Autodesk Inventor part; units mm, degrees
ref_plane "YZ Plane" through (0, 0, 0) normal (1, 0, 0) x (0, 1, 0)
ref_plane "XZ Plane" through (0, 0, 0) normal (0, 1, 0) x (-1, 0, 0)
ref_plane "XY Plane" through (0, 0, 0) normal (0, 0, 1) x (1, 0, 0)
sketch "Sketch1" plane through (0, 0, 0) normal (0, 1, 0) x (-1, 0, 0)
  line L0 (10, -18.5) -> (-10, -18.5)
  line L1 (-10, -18.5) -> (-10, 18.5)
  line L2 (-10, 18.5) -> (10, 18.5)
  line L3 (10, 18.5) -> (10, -18.5)
  point P0 (0, 0)
  dimension "d0" = 20
  dimension "d1" = 37
  dimension "d2" = 18.5
  dimension "d3" = 10
extrude "Plate1" add sketch "Sketch1" along normal blind 1.5
sketch "Sketch2" plane through (-10, 0, -20) normal (0, 0, 1) x (1, 0, 0)
  line L0 (20, 0) -> (0, 0)
  line L1 (0, 0) -> (0, 31.5)
  line L2 (0, 31.5) -> (20, 31.5)
  line L3 (20, 31.5) -> (20, 0)
edge flange "Flange1" height 31.5 angle 90 thickness 1.5 bend radius 0.31 thickness toward (0, 0, 1) relief tear relief width 1.5 relief depth 0.75 edges at (0, 1.5, -18.5) wall of the first edge with corners at (10, 0, -20) (-10, 0, -20) (-10, 31.5, -20) (10, 31.5, -20)
bend "Bend1"
corner "Corner1"
sketch "Sketch3" plane through (10, 0, 20) normal (0, 0, -1) x (-1, 0, 0)
  line L0 (20, 0) -> (0, 0)
  line L1 (0, 0) -> (0, 51.5)
  line L2 (0, 51.5) -> (20, 51.5)
  line L3 (20, 51.5) -> (20, 0)
edge flange "Flange2" height 51.5 angle 90 thickness 1.5 bend radius 0.31 thickness toward (0, 0, -1) relief tear relief width 1.5 relief depth 0.75 edges at (0, 1.5, 18.5) wall of the first edge with corners at (-10, 0, 20) (10, 0, 20) (10, 51.5, 20) (-10, 51.5, 20)
bend "Bend2"
corner "Corner2"
sketch "Sketch4" plane through (-10, 51.5, 20) normal (0, 0, 1) x (1, 0, 0)
  circle A0 centre (10, -10) radius 10
  line L0 (0, 0) -> (20, 0)
  line L1 (0, 0) -> (20, 0)
  line L2 (20, 0) -> (20, -10)
  line L3 (20, -10) -> (0, -10)
  line L4 (0, -10) -> (0, 0)
  line L5 (0, -49.69) -> (0, 0)
  point P0 (10, -51.5)
  point P1 (10, 0)
  dimension "d26" = 20
  dimension "d25" = 10
  dimension "d27" = 10
  dimension "d28" = 10
extrude "Extrusion1" cut sketch "Sketch4" against normal blind 10 contours L4 L0 A0 | A0 L0 L2
equation "\"d4\" = Thickness"
equation "\"d5\" = BendReliefWidth"
equation "\"d6\" = BendReliefDepth"
equation "\"d7\" = MinimumRemnant"
equation "\"d8\" = TransitionRadius"
equation "\"d11\" = BendRadius"
equation "\"d12\" = CornerReliefSize"
equation "\"d13\" = GapSize"
equation "\"d14\" = JacobiRadiusSize"
equation "\"d15\" = BendReliefWidth"
equation "\"d16\" = BendReliefDepth"
equation "\"d17\" = MinimumRemnant"
equation "\"d18\" = TransitionRadius"
equation "\"d21\" = BendRadius"
equation "\"d22\" = CornerReliefSize"
equation "\"d23\" = GapSize"
equation "\"d24\" = JacobiRadiusSize"
equation "\"BendReliefWidth\" = Thickness"
equation "\"BendReliefDepth\" = 0.5 * Thickness"
equation "\"CornerReliefSize\" = 4 * Thickness"
equation "\"MinimumRemnant\" = 2 * Thickness"
equation "\"TransitionRadius\" = BendRadius"
equation "\"JacobiRadiusSize\" = BendRadius"
equation "\"GapSize\" = Thickness"
properties part number "axis_9_bottom_frame" material "Aluminum 6061-AHC"
Design review of the part built by this model. Coordinates are the model's own, in mm. A direction names the side the tool comes from. Coordinates: 2 decimals unless noted, no trailing zeros. Order: outer loops, then holes, each group sorted by start corner. A loop starts at its lowest first (then second) coordinate and runs counter-clockwise, first axis right, second up. Notation, with made-up numbers: (63.25, 55.5) - (88.25, 55.5) arc R14 ccw to (88.25, 75.5) - close; hole circle Ø7 at (36, 28.25). An arc over 180 degrees is marked (long way). Answer in a Markdown table with one row per item.
(1) Consider section A-A on y = 22.5. State the section outline as (x, z) points.
Checked values:
| item | result |
|---|---|
| outline | (-10, -20) - (10, -20) - (10, -18.5) - (-10, -18.5) - close; (-10, 18.5) - (10, 18.5) - (10, 20) - (-10, 20) - close |
(2) The part is to be moulded in two halves that separate along Z. For faces 1 (the flat face through (0, 1.5, 0)), 2 (the cylindrical face through (-0.14, 0.54, -19.48)), 3 (the flat face through (0, 26, 18.5)), 4 (the cylindrical face through (0.14, 0.54, 19.48)), say which applies: released by +Z, released by -Z, zero draft, split by the parting line, or undercut.
Checked values:
| item | result |
|---|---|
| face 1 | undercut |
| face 2 | released by -Z |
| face 3 | undercut |
| face 4 | released by +Z |
(3) Consider section B-B on x = 0. State the section outline as (y, z) points, plus the area to 3 significant figures.
Checked values:
| item | result |
|---|---|
| outline | (0, -18.19) arc R1.81 ccw to (1.81, -20) - (31.5, -20) - (31.5, -18.5) - (1.81, -18.5) arc R0.31 cw to (1.5, -18.19) - (1.5, 18.19) arc R0.31 cw to (1.81, 18.5) - (51.5, 18.5) - (51.5, 20) - (1.81, 20) arc R1.81 ccw to (0, 18.19) - close |
| area | 179 mm^2 |
(4) Wall thickness on line 1 along Z through (x, y) = (-8.5, 15); line 2 along Y through (x, z) = (-3, 12.5); line 3 along Z through (x, y) = (1.75, 42.5): over which ranges is each line inside the solid? List them lowest first. Write a range as from..to.
Checked values:
| item | result |
|---|---|
| line 1 | -20..-18.5, 18.5..20 |
| line 2 | 0..1.5 |
| line 3 | 18.5..20 |
(5) Consider section D-D on y = 33. State the section outline as (x, z) points, plus the area to 3 significant figures.
Checked values:
| item | result |
|---|---|
| outline | (-10, 18.5) - (10, 18.5) - (10, 20) - (-10, 20) - close |
| area | 30.0 mm^2 |
(6) Clearance check with flat-ended pins moving along their axes: pin 1 (1.2 mm diameter, centred on x = 1, z = -19.5, fed in from +Y); pin 2 (3 mm diameter, centred on x = 0, y = 35.5, fed in from -Z); pin 3 (6 mm diameter, centred on x = 1.5, z = 6.5, fed in from +Y). State where each tip first meets the part, or that it passes through.
Checked values:
| item | result |
|---|---|
| pin 1 | y = 31.5 |
| pin 2 | z = 18.5 |
| pin 3 | y = 1.5 |
(7) For faces 5 (the flat face through (0, 16, -18.5)), 6 (the flat face through (0, 27, 20)), 7 (the flat face through (0, 31.5, -19)), list the 3-axis set-ups (+Z, -Z, +X, -X, +Y, -Y) from which the entire face can be reached by the end or side of a thin tool; tool diameter is ignored.
Checked values:
| item | result |
|---|---|
| face 5 | +X, -X, +Y |
| face 6 | +Z, +X, -X, +Y, -Y |
| face 7 | -Z, +X, -X, +Y |
(8) Consider section C-C on z = -14.5. State the section outline as (x, y) points, plus the area to 3 significant figures.
Checked values:
| item | result |
|---|---|
| outline | (-10, 0) - (10, 0) - (10, 1.5) - (-10, 1.5) - close |
| area | 30.0 mm^2 |
